```python
from build123d import *

# Parameters (mm, degrees)
F0_W     = 18
F0_H     = 22
F1_DEPTH = 7
F2_DEPTH = 3
F3_DEPTH = 3
F4_DEPTH = 25


with BuildPart() as f1:
    # F0 (on Top) → F1 (new body)
    with BuildSketch(Plane.XY):
        Polygon((15, 5), (15, 15), (10, 15), (5, 15), (-5, 15), (-10, 15), (-15, 15), (-15, 5), (-15, -15), (15, -15), align=None)
        Rectangle(F0_W, F0_H, mode=Mode.SUBTRACT)
    extrude(amount=F1_DEPTH)

    # F0 (on Top) → F2 (join)
    with BuildSketch(Plane.XY):
        Rectangle(F0_W, F0_H)
        with BuildLine():
            ThreePointArc((2.5, 2.927883), (3.496248, 1.612064), (3.85, 0))
            ThreePointArc((3.85, 0), (3.496248, -1.612064), (2.5, -2.927883))
            Line((2.5, -2.927883), (2.5, -6))
            Line((2.5, -6), (-2.5, -6))
            Line((-2.5, -6), (-2.5, -2.927883))
            ThreePointArc((-2.5, -2.927883), (-3.85, 0), (-2.5, 2.927883))
            Line((-2.5, 2.927883), (-2.5, 6))
            Line((-2.5, 6), (2.5, 6))
            Line((2.5, 6), (2.5, 2.927883))
        make_face(mode=Mode.SUBTRACT)
    extrude(amount=F2_DEPTH)

    # F0 (on Top) → F3 (join)
    with BuildSketch(Plane.XY):
        with BuildLine():
            Line((-15, 15), (-10, 15))
            Line((-10, 15), (-43.230891, 72.557591))
            ThreePointArc((-43.230891, 72.557591), (-48.26689, 71.973599), (-53.295612, 71.329946))
            Line((-53.295612, 71.329946), (-15, 5))
            Line((-15, 5), (-15, 15))
        make_face()
        with BuildLine():
            Line((-5, 15), (5, 15))
            Line((5, 15), (21.013009, 74.761364))
            ThreePointArc((21.013009, 74.761364), (16.540642, 74.921132), (12.066847, 75.034088))
            Line((12.066847, 75.034088), (0, 30))
            Line((0, 30), (-12.014256, 74.837814))
            ThreePointArc((-12.014256, 74.837814), (-16.469144, 74.652721), (-20.92186, 74.42119))
            Line((-20.92186, 74.42119), (-5, 15))
        make_face()
        with BuildLine():
            Line((10, 15), (15, 15))
            Line((15, 15), (15, 5))
            Line((15, 5), (53.772336, 72.155656))
            ThreePointArc((53.772336, 72.155656), (48.700199, 72.725298), (43.621624, 73.234362))
            Line((43.621624, 73.234362), (10, 15))
        make_face()
    extrude(amount=F3_DEPTH)

    # F0 (on Top) → F4 (join)
    with BuildSketch(Plane.XY):
        with BuildLine():
            ThreePointArc((21.013009, 74.761364), (32.327433, 74.147641), (43.621624, 73.234362))
            ThreePointArc((43.621624, 73.234362), (48.700199, 72.725298), (53.772336, 72.155656))
            ThreePointArc((53.772336, 72.155656), (59.070627, 71.495011), (64.360257, 70.768265))
            Line((64.360257, 70.768265), (64.360257, 75.768265))
            ThreePointArc((64.360257, 75.768265), (-0.734726, 85.130056), (-65.633486, 74.49281))
            Line((-65.633486, 74.49281), (-65.633486, 69.49281))
            ThreePointArc((-65.633486, 69.49281), (-59.471248, 70.456366), (-53.295612, 71.329946))
            ThreePointArc((-53.295612, 71.329946), (-48.26689, 71.973599), (-43.230891, 72.557591))
            ThreePointArc((-43.230891, 72.557591), (-32.088572, 73.6354), (-20.92186, 74.42119))
            ThreePointArc((-20.92186, 74.42119), (-16.469144, 74.652721), (-12.014256, 74.837814))
            ThreePointArc((-12.014256, 74.837814), (0.024914, 75.105497), (12.066847, 75.034088))
            ThreePointArc((12.066847, 75.034088), (16.540642, 74.921132), (21.013009, 74.761364))
        make_face()
    extrude(amount=F4_DEPTH)


solid = f1.part
```
Design review of the part built by this model. Coordinates are the model's own, in mm. A direction names the side the tool comes from. Coordinates: 2 decimals unless noted, no trailing zeros. Loops run counter-clockwise (first coordinate to the right, second up) from the corner with the lowest first, then second, coordinate; pieces in that order, holes last. Notation, with made-up numbers: (-18, 31.25) - (38, 31.25) arc R29 cw to (38, 59.25) - close; hole circle Ø6 at (-38, 52.25). An arc over 180 degrees is marked (long way). Use CSV: the item, a comma, the result in double quotes. Start each with the question number.
1) Consider section D-D on y = 1.5. Write out the cut boundary in (x, z), then the cut area to 3 significant figures.
2) Consider section A-A on x = -25.5. Write out the cut boundary in (y, z).
3) For pin 1 Ø1.5 at (x, z) = (-30.5, 6.5) entering from -Y; pin 2 Ø21.5 at (x, y) = (-39.5, 44) entering from +Z; pin 3 Ø2 at (y, z) = (5.5, 4.5) entering from -X, all flat-tipped, find the tip position at first contact; note any pin that passes through.
4) The part is to be moulded in two halves that separate along X. For faces 1 (the flat face through (2.5, 4, 1)), 2 (the flat face through (15, -4, 3)), 3 (the flat face through (-2, 77, 25)), say which applies: +X half, -X half, draft (parallel to the pull), parting line (faces both ways), or undercut.
5) Tool access review of faces 4 (the cylindrical face through (58.997, 71.505, 12.325)), 5 (the flat face through (9, 0, 5)), 6 (the flat face through (-26.383, 43.376, 1.479)): name each direction out of +Z, -Z, +X, -X, +Y, -Y from which nothing blocks a thin tool from reaching the whole face with its end or side.
6) Consider section B-B on y = 66. Write out the cut boundary in (x, z), then the cut area to 3 significant figures.
7) Wall thickness on L1, parallel to Z at x = -17, y = 67; L2, parallel to X at y = -1.5, z = 2.5; L3, parallel to Y at x = 20.5, z = 8.25: over which ranges is each line inside the solid? List them lowest first. Write a range as from..to.
8) Consider section C-C on z = 21.5. Write out the cut boundary in (x, y).
Geometry says:
1,outline,"(-15, 0) - (-3.55, 0) - (-3.55, 3) - (-9, 3) - (-9, 7) - (-15, 7) - close; (3.55, 0) - (15, 0) - (15, 7) - (9, 7) - (9, 3) - (3.55, 3) - close"
1,area,"117 mm^2"
2,outline,"(23.19, 0) - (41.85, 0) - (41.85, 3) - (23.19, 3) - close; (74.13, 0) - (83.46, 0) - (83.46, 25) - (74.13, 25) - close"
3,pin 1,"y = 73.7"
3,pin 2,"z = 3"
3,pin 3,"x = -15"
4,face 1,"undercut"
4,face 2,"+X half"
4,face 3,"draft"
5,face 4,"+Z, -Z, -Y"
5,face 5,"+Z"
5,face 6,"+Z, -Z"
6,outline,"(-50.22, 0) - (-39.44, 0) - (-39.44, 3) - (-50.22, 3) - close; (-18.67, 0) - (-9.65, 0) - (-9.65, 3) - (-18.67, 3) - close; (9.65, 0) - (18.67, 0) - (18.67, 3) - (9.65, 3) - close; (39.44, 0) - (50.22, 0) - (50.22, 3) - (39.44, 3) - close"
6,area,"119 mm^2"
7,L1,"0..3"
7,L2,"-15..-3.55, 3.55..15"
7,L3,"74.78..84.29"
8,outline,"(-65.63, 69.49) arc R427.64 cw to (-53.3, 71.33) arc R427.64 cw to (-43.23, 72.56) arc R427.64 cw to (-20.92, 74.42) arc R427.64 cw to (-12.01, 74.84) arc R427.64 cw to (12.07, 75.03) arc R427.63 cw to (21.01, 74.76) arc R427.64 cw to (43.62, 73.23) arc R427.63 cw to (53.77, 72.16) arc R427.63 cw to (64.36, 70.77) - (64.36, 75.77) arc R216.25 ccw to (-65.63, 74.49) - close"
